The listing builds one solid part. Answer for the finished solid, in the listing's coordinates (mm). Face numbers are marked on the shaded views. Round coordinates to 2 decimals unless told otherwise and drop trailing zeros. Write each loop counter-clockwise with the first axis right and the second up, starting at its lowest first coordinate (ties: lowest second). Pieces come first, ordered by that corner, then holes. Notation, with made-up numbers: M 28,37 L 32,37 A16 cw 32,64 Z; hole C 43,62 d5. An arc over 180 degrees is marked long. Write each question's results on one line, items separated by ' | '.
Autodesk Inventor part; units mm, degrees
ref_plane "YZ Plane" through (0, 0, 0) normal (1, 0, 0) x (0, 1, 0)
ref_plane "XZ Plane" through (0, 0, 0) normal (0, 1, 0) x (-1, 0, 0)
ref_plane "XY Plane" through (0, 0, 0) normal (0, 0, 1) x (1, 0, 0)
sketch "Sketch1" plane through (0, 0, 0) normal (0, 0, 1) x (1, 0, 0)
  circle A0 centre (0, 0) radius 457.2
  circle A1 centre (0, 0) radius 444.5
  dimension "d0" = 914.4
  dimension "d1" = 889
extrude "Extrusion1" add sketch "Sketch1" along normal blind 369.0375
chamfer "Chamfer1" distance 11.1125 angle 37.5 1 edges at (-457.2, 0, 0) measured on face at (-448.3191, -14.9353, 0)
chamfer "Chamfer2" distance 11.1125 angle 37.5 1 edges at (-457.2, 0, 369.0375) measured on face at (-448.3191, -14.9353, 369.0375)
equation "\"d7\" = d4"
equation "\"d9\" = d6"
properties part number "A1-19027-100-02 36in pipe" material "Steel, Mild"
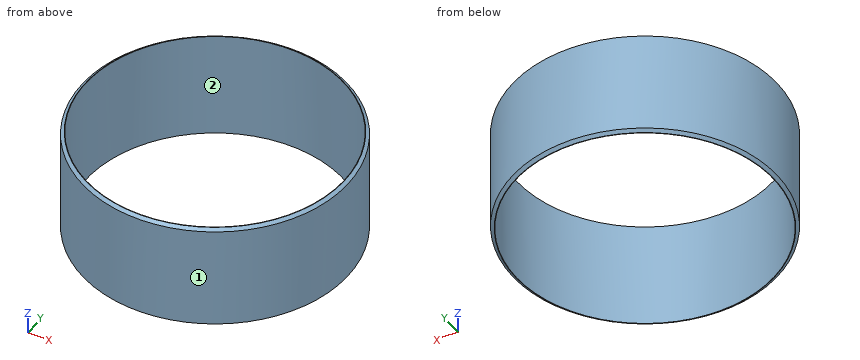
1) Section C-C (z = 189) is taken. Determine the outline of the cut face in (x, y).
Return value:
outline: C 0,0 d914.4; hole C 0,0 d889
2) Section A-A (x = 0) is taken. Determine the outline of the cut face in (y, z), then the cut area to 3 significant figures.
Return value:
outline: M -457.2,8.53 L -446.09,0 L -444.5,0 L -444.5,369.04 L -446.09,369.04 L -457.2,360.51 Z; M 444.5,0 L 446.09,0 L 457.2,8.53 L 457.2,360.51 L 446.09,369.04 L 444.5,369.04 Z | area: 9,180 mm²
3) Each of these flat-tipped pins is pushed along its axis until it touches: pin 1 (8 mm diameter, centred on x = -287, z = 80.5, fed in from -Y); pin 2 (6 mm diameter, centred on x = 283.5, z = 239, fed in from -Y); pin 3 (1 mm diameter, centred on x = -313.5, z = 253, fed in from +Y). Where does it stop, or does it pass through?
Return value:
pin 1: y = -359.09 | pin 2: y = -361.04 | pin 3: y = 333.26
4) The mould has two halves that part along X. Classify the marked faces 1 and 2: +X half, -X half, draft (parallel to the pull), parting line (faces both ways), or undercut.
Return value:
face 1: parting line | face 2: undercut
5) Find the intervals of material crossed by line 1 (Y direction, x = -1.5, z = 290.5); line 2 (X direction, y = -88, z = 131.5); line 3 (X direction, y = -89, z = 227), in increasing order.
Return value:
line 1: -457.2 to -444.5, 444.5 to 457.2 | line 2: -448.65 to -435.7, 435.7 to 448.65 | line 3: -448.45 to -435.5, 435.5 to 448.45
